Model file for the job. Use its own axes, mm. Give positions to 0.01 mm unless a question says otherwise; leave off trailing zeros. Loops run counter-clockwise (first coordinate to the right, second up) from the corner with the lowest first, then second, coordinate; pieces in that order, holes last. Notation, with made-up numbers: M 20.5,45.25 L 78.5,45.25 A12 cw 78.5,60.25 Z; hole C 49.25,-36.5 d3. An arc over 180 degrees is marked long. Answer in a Markdown table with one row per item.
```python
from build123d import *

# Parameters (mm, degrees)
SKETCH_1_W          = 20
SKETCH_1_H          = 420
EXTRUDE_1_DEPTH     = 5
SKETCH_2_R          = 1.5
CUT_EXTRUDE_1_DEPTH = 211.297408448
SKETCH_3_W          = 10
SKETCH_3_H          = 35
CUT_EXTRUDE_2_DEPTH = 211.297408448
FILLET_1_R          = 3


with BuildPart() as part:
    # 草图1 → 凸台-拉伸1 (new body)
    with BuildSketch(Plane(origin=(0, 0, 0), x_dir=(1, 0, 0), z_dir=(0, 1, 0))):
        Rectangle(SKETCH_1_W, SKETCH_1_H)
    extrude(amount=EXTRUDE_1_DEPTH)

    # 草图2 → 切除-拉伸1 (cut, through all)
    with BuildSketch(Plane(origin=(0, 5, 0), x_dir=(1, 0, 0), z_dir=(0, 1, 0))):
        with Locations(Location((0, 0, 0), (0, 0, 270))):
            Circle(SKETCH_2_R)
        with Locations(Location((0, 50, 0), (0, 0, 270))):
            Circle(SKETCH_2_R)
        with Locations(Location((0, 100, 0), (0, 0, 270))):
            Circle(SKETCH_2_R)
        with Locations(Location((0, 150, 0), (0, 0, 270))):
            Circle(SKETCH_2_R)
        with Locations(Location((0, 200, 0), (0, 0, 270))):
            Circle(SKETCH_2_R)
        with Locations(Location((0, -200, 0), (0, 0, 90))):
            Circle(SKETCH_2_R)
        with Locations(Location((0, -150, 0), (0, 0, 90))):
            Circle(SKETCH_2_R)
        with Locations(Location((0, -100, 0), (0, 0, 90))):
            Circle(SKETCH_2_R)
        with Locations(Location((0, -50, 0), (0, 0, 90))):
            Circle(SKETCH_2_R)
    extrude(amount=-CUT_EXTRUDE_1_DEPTH, mode=Mode.SUBTRACT)

    # 草图3 → 切除-拉伸2 (cut, through all)
    with BuildSketch(Plane(origin=(0, 5, 0), x_dir=(1, 0, 0), z_dir=(0, 1, 0))):
        with Locations((0, 125)):
            Rectangle(SKETCH_3_W, SKETCH_3_H)
        with Locations((0, 175)):
            Rectangle(SKETCH_3_W, SKETCH_3_H)
        with Locations((0, 75)):
            Rectangle(SKETCH_3_W, SKETCH_3_H)
        with Locations((0, 25)):
            Rectangle(SKETCH_3_W, SKETCH_3_H)
        with Locations((0, -25)):
            Rectangle(SKETCH_3_W, SKETCH_3_H)
        with Locations((0, -75)):
            Rectangle(SKETCH_3_W, SKETCH_3_H)
        with Locations((0, -125)):
            Rectangle(SKETCH_3_W, SKETCH_3_H)
        with Locations((0, -175)):
            Rectangle(SKETCH_3_W, SKETCH_3_H)
    extrude(amount=-CUT_EXTRUDE_2_DEPTH, mode=Mode.SUBTRACT)

    # 圆角1
    fillet_1_edges = [part.edges().sort_by_distance(p)[0] for p in [
        (-5, 2.5, -42.5),
        (5, 2.5, -42.5),
        (5, 2.5, -7.5),
        (-5, 2.5, -7.5),
        (-5, 2.5, 7.5),
        (5, 2.5, 7.5),
        (5, 2.5, 42.5),
        (-5, 2.5, 42.5),
        (-5, 2.5, 57.5),
        (5, 2.5, 57.5),
        (5, 2.5, 92.5),
        (-5, 2.5, 92.5),
        (-5, 2.5, 107.5),
        (5, 2.5, 107.5),
        (5, 2.5, 142.5),
        (-5, 2.5, 142.5),
        (-5, 2.5, 157.5),
        (5, 2.5, 157.5),
        (5, 2.5, 192.5),
        (-5, 2.5, 192.5),
        (5, 2.5, -192.5),
        (5, 2.5, -157.5),
        (-5, 2.5, -157.5),
        (-5, 2.5, -192.5),
        (-5, 2.5, -142.5),
        (5, 2.5, -142.5),
        (5, 2.5, -107.5),
        (-5, 2.5, -107.5),
        (-5, 2.5, -92.5),
        (5, 2.5, -92.5),
        (5, 2.5, -57.5),
        (-5, 2.5, -57.5),
    ]]
    fillet(fillet_1_edges, radius=FILLET_1_R)


solid = part.part
```
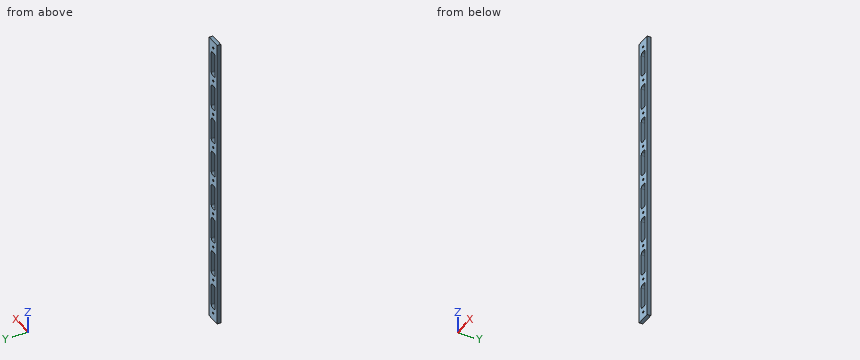
Q1. Probe probe 1 along X at (y, z) = (3.4, 163.5); probe 2 along X at (y, z) = (2.05, 150). List the from-to ranges inside material, lowest first.
Reported:
| item | result |
|---|---|
| probe 1 | -10 to -5, 5 to 10 |
| probe 2 | -10 to -1.5, 1.5 to 10 |
Q2. Saw through at A-A (z = 19). Give the cut face in (x, y).
Reported:
| item | result |
|---|---|
| outline | M -10,0 L -5,0 L -5,5 L -10,5 Z; M 5,0 L 10,0 L 10,5 L 5,5 Z |
Q3. Saw through at B-B (y = 1.45). Give the number of separate pieces and of enclosed holes in the cut face, and give its area (3 significant figures).
Reported:
| item | result |
|---|---|
| separate pieces | 1 |
| enclosed holes | 17 |
| area | 5,600 mm² |
